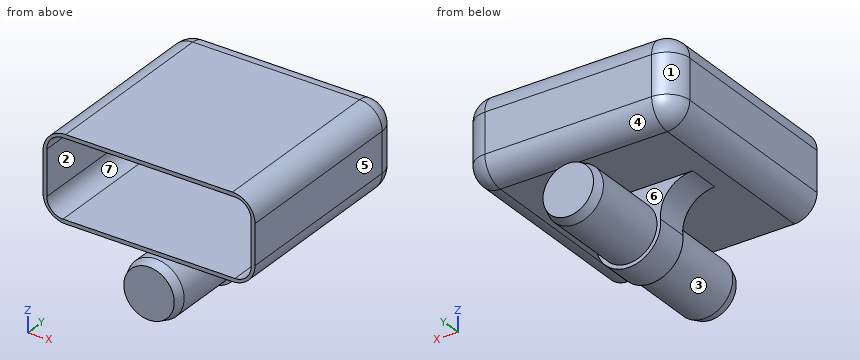
Autodesk Inventor part; units mm, degrees
ref_plane "YZ Plane" through (0, 0, 0) normal (1, 0, 0) x (0, 1, 0)
ref_plane "XZ Plane" through (0, 0, 0) normal (0, 1, 0) x (-1, 0, 0)
ref_plane "XY Plane" through (0, 0, 0) normal (0, 0, 1) x (1, 0, 0)
sketch "Sketch1" plane through (0, 0, 0) normal (0, 1, 0) x (-1, 0, 0)
  line L0 (3.8011, 12.3974) -> (-61.8989, 12.3974)
  line L1 (-61.8989, 12.3974) -> (-61.8989, -14.0026)
  line L2 (-61.8989, -14.0026) -> (3.8011, -14.0026)
  line L3 (3.8011, -14.0026) -> (3.8011, 12.3974)
  line L4 (2.6011, 11.1974) -> (-60.6989, 11.1974)
  line L5 (-60.6989, 11.1974) -> (-60.6989, -12.8026)
  line L6 (-60.6989, -12.8026) -> (2.6011, -12.8026)
  line L7 (2.6011, -12.8026) -> (2.6011, 11.1974)
  point P0 (0, 0)
  dimension "d0" = 26.4
  dimension "d1" = 65.7
  dimension "d2" = 1.2
  dimension "d3" = 24
  dimension "d4" = 63.3
extrude "Extrusion1" add sketch "Sketch1" along normal blind 1.2 contours L3 L2 L1 L0 | L7 L6 L5 L4
extrude "Extrusion2" add sketch "Sketch1" against normal blind 63
fillet "Fillet1" radius 5 8 edges at (29.0489, 0, 11.1974) (-2.6011, -31.5, 11.1974) (-2.6011, 0, -0.8026) (29.0489, 0, -12.8026) (60.6989, 0, -0.8026) (60.6989, -31.5, -12.8026) (-2.6011, -31.5, -12.8026) (60.6989, -31.5, 11.1974)
ref_plane "Work Plane1" through (0, -30.9, 0) normal (0, 1, 0) x (1, 0, 0)
sketch "Sketch3" plane through (0, -30.9, 0) normal (0, 1, 0) x (1, 0, 0)
  arc A0 (2.3989, 12.8026) -> (-2.6011, 7.8026) centre (2.3989, 7.8026) ccw
  line L0 (-2.6011, 7.8026) -> (-2.6011, -6.1974)
  arc A1 (-2.6011, -6.1974) -> (2.3989, -11.1974) centre (2.3989, -6.1974) ccw
  line L1 (2.3989, -11.1974) -> (55.6989, -11.1974)
  arc A2 (55.6989, -11.1974) -> (60.6989, -6.1974) centre (55.6989, -6.1974) ccw
  line L2 (60.6989, -6.1974) -> (60.6989, 7.8026)
  arc A3 (60.6989, 7.8026) -> (55.6989, 12.8026) centre (55.6989, 7.8026) ccw
  line L3 (55.6989, 12.8026) -> (2.3989, 12.8026)
  line L4 (61.8989, -12.3974) -> (-3.8011, -12.3974)
  line L5 (-3.8011, -12.3974) -> (-3.8011, 14.0026)
  line L6 (-3.8011, 14.0026) -> (61.8989, 14.0026)
  line L7 (61.8989, 14.0026) -> (61.8989, -12.3974)
  circle A4 centre (29.0489, 26.0026) radius 8.825
  circle A5 centre (29.0489, 26.0026) radius 10
  circle A6 centre (9.1492, 24.0026) radius 10
  circle A7 centre (48.9487, 24.0026) radius 10
  point P0 (0, 0)
  point P1 (29.0489, 14.0026)
  point P2 (48.9487, 14.0026)
  point P3 (38.9988, 25.0026)
  point P4 (19.099, 25.0026)
  point P5 (9.1492, 14.0026)
  dimension "d10" = 17.65
  dimension "d11" = 20
  dimension "d12" = 12
  dimension "d13" = 20
  dimension "d14" = 20
extrude "Extrusion3" add sketch "Sketch3" along normal mid plane 10 contours L6 A6 A5 A7 | A5 | A4
extrude "Extrusion4" add sketch "Sketch3" along normal mid plane 64.2 contours A4
chamfer "Chamfer1" distance 1 distance2 3 1 edges at (20.2239, -63, -26.0026) measured on face at (28.7756, -63, -23.412)
chamfer "Chamfer2" distance 1 distance2 3 1 edges at (20.2239, 1.2, -26.0026) measured on face at (28.7756, 1.2, -23.412)
fillet "Fillet2" radius 7 8 edges at (61.8989, -30.9, -14.0026) (61.8989, -30.9, 12.3974) (-3.8011, -30.9, 12.3974) (-3.8011, -30.9, -14.0026) (-3.8011, 1.2, -0.8026) (29.0489, 1.2, 12.3974) (61.8989, 1.2, -0.8026) (29.0489, 1.2, -14.0026)
properties part number "batteriehalter"
Could you check a few things on this model? Use its own coordinates, in mm. Face numbers are marked on the shaded views. A direction names the side the tool comes from. Round coordinates to 2 decimals unless told otherwise and drop trailing zeros. Loops run counter-clockwise (first coordinate to the right, second up) from the corner with the lowest first, then second, coordinate; pieces in that order, holes last. Notation, with made-up numbers: (41, 39) - (58, 39) arc R5 cw to (58, 43) - close; hole circle Ø1 at (32.5, 51). An arc over 180 degrees is marked (long way). Answer in a Markdown table with one row per item. Add a question column.
(1) If we section it at C-C (z = -3): Please give me the cut outline in (x, y).
(2) If we section it at A-A (y = -47.5): Please give me the cut outline in (x, z) (3 decimals).
(3) If we section it at D-D (y = -4): Please give me the cut outline in (x, z) (3 decimals).
(4) I'm going to push flat-ended pins straight in: pin 1 (5 mm diameter, centred on x = 52.5, y = -34, fed in from -Z); pin 2 (1.5 mm diameter, centred on x = 13, z = 3.5, fed in from -Y); pin 3 (6 mm diameter, centred on y = -44, z = -11.5, fed in from -X). Where does each tip first touch, or does it pass through?
(5) I need wall thicknesses on line 1 along X through (y, z) = (-56.5, 1.5); line 2 along Z through (x, y) = (43, -52.5); line 3 along Z through (x, y) = (36.5, -49). Which ranges of each line are inside material? Lowest first, please.
(6) If we mould it in two halves opening along X, with no side actions, what happens to the marked faces 1, 2 and 3? For each: pulls with the +X half, pulls with the -X half, needs draft (parallel to the pull), parting line crosses it, or undercut.
(7) If we section it at B-B (x = 42): Please give me the cut outline in (y, z).
(8) For the marked faces 4, 5, 6 and 7, which set-ups out of +Z, -Z, +X, -X, +Y, -Y let a thin tool reach every point of the face, with its end or its side?
Model answer:
| question | item | result |
|---|---|---|
| 1 | outline | (-3.8, -63) - (-2.6, -63) - (-2.6, -5) arc R5 cw to (2.4, 0) - (55.7, 0) arc R5 cw to (60.7, -5) - (60.7, -63) - (61.9, -63) - (61.9, -5.8) arc R7 ccw to (54.9, 1.2) - (3.2, 1.2) arc R7 ccw to (-3.8, -5.8) - close |
| 2 | outline | (-3.801, -7.003) arc R7 ccw to (3.199, -14.003) - (54.899, -14.003) arc R7 ccw to (61.899, -7.003) - (61.899, 5.397) arc R7 ccw to (54.899, 12.397) - (3.199, 12.397) arc R7 ccw to (-3.801, 5.397) - close; circle Ø17.65 at (29.049, -26.003); hole (-2.601, -7.803) arc R5 ccw to (2.399, -12.803) - (55.699, -12.803) arc R5 ccw to (60.699, -7.803) - (60.699, 6.197) arc R5 ccw to (55.699, 11.197) - (2.399, 11.197) arc R5 ccw to (-2.601, 6.197) - close |
| 3 | outline | (-3.566, -7.003) arc R6.765 ccw to (3.199, -13.767) - (54.899, -13.767) arc R6.765 ccw to (61.664, -7.003) - (61.664, 5.397) arc R6.765 ccw to (54.899, 12.162) - (3.199, 12.162) arc R6.765 ccw to (-3.566, 5.397) - close; circle Ø17.65 at (29.049, -26.003); hole (-2.5, -7.803) arc R4.899 ccw to (2.399, -12.702) - (55.699, -12.702) arc R4.899 ccw to (60.598, -7.803) - (60.598, 6.197) arc R4.899 ccw to (55.699, 11.096) - (2.399, 11.096) arc R4.899 ccw to (-2.5, 6.197) - close |
| 4 | pin 1 | stops at z = -14 |
| 4 | pin 2 | stops at y = 0 |
| 4 | pin 3 | stops at x = -3.64 |
| 5 | line 1 | x = -3.8 to -2.6, 60.7 to 61.9 |
| 5 | line 2 | z = -14 to -12.8, 11.2 to 12.4 |
| 5 | line 3 | z = -30.73 to -21.27, -14 to -12.8, 11.2 to 12.4 |
| 6 | face 1 | pulls with the -X half |
| 6 | face 2 | undercut |
| 6 | face 3 | parting line crosses it |
| 7 | outline | (-63, -14) - (-35.9, -14) - (-35.9, -16.81) - (-25.9, -16.81) - (-25.9, -14) - (-5.8, -14) arc R7 ccw to (1.2, -7) - (1.2, 5.4) arc R7 ccw to (-5.8, 12.4) - (-63, 12.4) - (-63, 11.2) - (-5, 11.2) arc R5 cw to (0, 6.2) - (0, -7.8) arc R5 cw to (-5, -12.8) - (-63, -12.8) - close |
| 8 | face 4 | +X, -X, +Y |
| 8 | face 5 | +Z, -Z, +X, +Y, -Y |
| 8 | face 6 | +Y |
| 8 | face 7 | -Y |
